from build123d import *

# Parameters (mm, degrees)
F0_R     = 52.5
F0_R_2   = 50.5
F1_DEPTH = 4
F2_W     = 2
F2_H     = 51.4
F2_W_2   = 51.4
F2_H_2   = 2
F3_DEPTH = 95
F5_DEPTH = 20
F6_F1_R  = 1
F6_F2_R  = 1
F6_F3_R  = 0.9999
F7_R     = 0.99999


# Not quite as in the source:
# - a fillet or chamfer is up to 0.001 mm smaller than in the source, because OpenCascade refuses the exact size


with BuildPart() as f1:
    # F0 (on Top) → F1 (new body)
    with BuildSketch(Plane.XY):
        Circle(F0_R)
        Circle(F0_R_2, mode=Mode.SUBTRACT)
    extrude(amount=F1_DEPTH)

    # F2 (on Top) → F3 (join)
    with BuildSketch(Plane.XY):
        with Locations((0, -26.7)):
            Rectangle(F2_W, F2_H)
        with Locations((-26.7, 0)):
            Rectangle(F2_W_2, F2_H_2)
        Rectangle(F2_W, F2_H_2)
        with Locations((26.7, 0)):
            Rectangle(F2_W_2, F2_H_2)
        with Locations((0, 26.7)):
            Rectangle(F2_W, F2_H)
    extrude(amount=F3_DEPTH)

    # F4 (on Top) → F5 (join)
    with BuildSketch(Plane.XY):
        with BuildLine():
            Line((0, 0), (52.5, 0))
            ThreePointArc((52.5, 0), (37.1231060123, 37.1231060123), (0, 52.5))
            Line((0, 52.5), (0, 0))
        make_face()
    extrude(amount=F5_DEPTH)

    # F6: fillet of radius 1 on 13 edges, made by hand

    # F6_f1
    f6_f1_edges = [f1.edges().sort_by_distance(p)[0] for p in [
        (1, 1, 57.5),
        (26.7, 1, 20),
        (1, 26.7, 20),
        (-1, 1, 47.5),
        (1, -1, 47.5),
        (-1, -1, 47.5),
    ]]
    fillet(f6_f1_edges, radius=F6_F1_R)

    # F6_f2
    f6_f2_edges = [f1.edges().sort_by_distance(p)[0] for p in [
        (-27.2, 1, 95),
        (-35.7088924499, -35.7088924499, 4),
        (35.7088924499, -35.7088924499, 4),
        (-35.7088924499, 35.7088924499, 0),
        (-35.7088924499, 35.7088924499, 4),
        (-1.2928932188, 1.2928932188, 95),
    ]]
    fillet(f6_f2_edges, radius=F6_F2_R)

    # F6_f3 (radius 1 in the source; OpenCascade refuses exactly that, so slightly less here)
    f6_f3_edges = [f1.edges().sort_by_distance(p)[0] for p in [
        (1, 27.2, 95),
        (27.2, 1, 95),
        (1.2928932188, 1.2928932188, 95),
    ]]
    fillet(f6_f3_edges, radius=F6_F3_R)

    # F7 (radius 1 in the source; OpenCascade refuses exactly that, so slightly less here)
    f7_edges = [f1.edges().sort_by_distance(p)[0] for p in [
        (1, -27.2, 95),
        (-1, -27.2, 95),
        (-27.2, -1, 95),
        (27.2, -1, 95),
        (1.292893, -1.292893, 95),
        (-1.292893, -1.292893, 95),
    ]]
    fillet(f7_edges, radius=F7_R)


solid = f1.part
Read the model definition and answer for the solid it produces. Units are mm, in the model's axes. A direction names the side the tool comes from. Coordinates: 2 decimals unless noted, no trailing zeros. Loops run counter-clockwise (first coordinate to the right, second up) from the corner with the lowest first, then second, coordinate; pieces in that order, holes last. Notation, with made-up numbers: (2, -6) -> (6, -6) arc R33 cw to (6, 22) -> close; hole circle Ø3 at (89, -17.5). An arc over 180 degrees is marked (long way). Answer in a Markdown table with one row per item.
Item 1: A cutting plane is placed at A-A on z = 57.5. Determine the outline of the cut face in (x, y), plus the area to 3 significant figures.
Returned:
| item | result |
|---|---|
| outline | (-52.4, -1) -> (-2, -1) arc R1 cw to (-1, -2) -> (-1, -52.4) -> (1, -52.4) -> (1, -2) arc R1 cw to (2, -1) -> (52.4, -1) -> (52.4, 1) -> (2, 1) arc R1 cw to (1, 2) -> (1, 52.4) -> (-1, 52.4) -> (-1, 2) arc R1 cw to (-2, 1) -> (-52.4, 1) -> close |
| area | 416 mm^2 |
Item 2: Straight lines are drawn through the part: line 1 along Y through (x, z) = (-14, 49.5); line 2 along Z through (x, y) = (36.5, 28.5). For each, find the intervals that lie inside material, in ascending order. Write a range as [from, to].
Returned:
| item | result |
|---|---|
| line 1 | y = [-1, 1] |
| line 2 | z = [0, 20] |
Item 3: Each of these flat-tipped pins is pushed along its axis until it touches: P1, Ø15, axis at x = -21, z = 60.5, coming from the +Y side; P2, Ø3.5, axis at x = 0, z = 35.5, coming from the +Y side; P3, Ø25, axis at y = -23.5, z = 39, coming from the +X side. Where does it stop, or does it pass through?
Returned:
| item | result |
|---|---|
| P1 | stops at y = 1 |
| P2 | stops at y = 52.4 |
| P3 | stops at x = 1 |
Item 4: For faces 5 (the flat face through (1, 27, 57)), 6 (the cylindrical face through (35.324, -36.09, 1.479)), 7 (the flat face through (-11.9, -50.3, 4)), determine the directions among +Z, -Z, +X, -X, +Y, -Y from which every point of the face is accessible in a straight line to the end or side of a thin tool.
Returned:
| item | result |
|---|---|
| face 5 | +Z, +X, +Y |
| face 6 | +Z, -Z |
| face 7 | +Z |
Item 5: A cutting plane is placed at B-B on x = -4. Give the number of separate pieces and of enclosed holes in the cut face, plus the area to 3 significant figures.
Returned:
| item | result |
|---|---|
| separate pieces | 3 |
| enclosed holes | 0 |
| area | 205 mm^2 |
Item 6: For a pull along Y with two mould halves and no side action, classify faces 1 (the cylindrical face through (50.076, 15.77, 5.416)), 2 (the flat face through (20, 21, 20)), 3 (the flat face through (0, 52.4, 49)), 4 (the cylindrical face through (-36.09, -35.324, 1.479)) as released by +Y, released by -Y, zero draft, split by the parting line, or undercut.
Returned:
| item | result |
|---|---|
| face 1 | split by the parting line |
| face 2 | zero draft |
| face 3 | released by +Y |
| face 4 | undercut |
Item 7: A cutting plane is placed at C-C on z = 9. Determine the outline of the cut face in (x, y).
Returned:
| item | result |
|---|---|
| outline | (-52.4, -1) -> (-2, -1) arc R1 cw to (-1, -2) -> (-1, -52.4) -> (1, -52.4) -> (1, -2) arc R1 cw to (2, -1) -> (52.4, -1) -> (52.4, 0) -> (52.5, 0) arc R52.5 ccw to (0, 52.5) -> (0, 52.4) -> (-1, 52.4) -> (-1, 2) arc R1 cw to (-2, 1) -> (-52.4, 1) -> close |
